Read the model definition and answer for the solid it produces. Units are mm, in the model's axes. Coordinates: 2 decimals unless noted, no trailing zeros. Write each loop counter-clockwise with the first axis right and the second up, starting at its lowest first coordinate (ties: lowest second). Pieces come first, ordered by that corner, then holes.
Item 1: Section C-C (z = -3.5) is taken. State how many separate pieces and enclosed holes the cut face has, then the cut area to 3 significant figures.
Item 2: Section B-B (y = -86.5) is taken. Give the vertices of the cut face in (x, z), then the cut area to 3 significant figures.
Item 3: Section A-A (x = 19) is taken. Give the vertices of the cut face in (y, z).
Item 4: Straight lines are drawn through the part: probe 1 along X at (y, z) = (-325, -0.25); probe 2 along Y at (x, z) = (475, -0.5); probe 3 along X at (y, z) = (-375, -1.5). For each, find the intervals that lie inside material, in ascending order.
Item 5: Each of these flat-tipped pins is pushed along its axis until it touches: P1, Ø3, axis at x = 466, z = 2, coming from the +Y side; P2, Ø3, axis at y = -371.5, z = -2, coming from the -X side; P3, Ø16.5, axis at x = -475, y = -325, coming from the +Z side; P4, Ø5, axis at y = 368.5, z = 0.5, coming from the +X side. Where does it stop, or does it pass through?
Autodesk Inventor part; units mm, degrees
ref_plane "YZ Plane" through (0, 0, 0) normal (1, 0, 0) x (0, 1, 0)
ref_plane "XZ Plane" through (0, 0, 0) normal (0, 1, 0) x (-1, 0, 0)
ref_plane "XY Plane" through (0, 0, 0) normal (0, 0, 1) x (1, 0, 0)
sketch "Sketch3" plane through (0, 0, 0) normal (0, 0, 1) x (1, 0, 0)
  line L0 (-500, -400) -> (500, -400)
  line L1 (500, -400) -> (500, 400)
  line L2 (500, 400) -> (-500, 400)
  line L3 (-500, 400) -> (-500, -400)
  line L4 (-500, -400) -> (500, 400) construction
  line L5 (500, -400) -> (-500, 400) construction
  point P0 (0, 0)
  dimension "d9" = 1000
  dimension "d10" = 800
extrude "Plate2" add sketch "Sketch3" along normal mid plane 10
sketch "Sketch4" plane through (0, 0, 5) normal (0, 0, 1) x (1, 0, 0)
  line L0 (-200, -175) -> (200, -175)
  line L1 (200, -175) -> (200, 175)
  line L2 (200, 175) -> (-200, 175)
  line L3 (-200, 175) -> (-200, -175)
  line L4 (-200, -175) -> (200, 175) construction
  line L5 (200, -175) -> (-200, 175) construction
  point P0 (0, 0)
  dimension "d12" = 400
  dimension "d13" = 350
extrude "Cut2" cut sketch "Sketch4" against normal blind 10
sketch "Sketch7" plane through (0, 0, 5) normal (0, 0, 1) x (1, 0, 0)
  line L0 (-450, 400) -> (-500, 400)
  line L1 (-500, 400) -> (-500, 350)
  line L2 (-500, 350) -> (-450, 350)
  line L3 (-450, 350) -> (-450, 400)
  line L4 (-450, 400) -> (-500, 350) construction
  line L5 (-500, 400) -> (-450, 350) construction
  circle A0 centre (-425, 375) radius 5.1
  circle A1 centre (-475, 325) radius 5.1
  point P0 (0, 0)
  point P1 (-475, 375)
  point P2 (-475, 375)
  point P3 (-475, 375)
  dimension "d20" = 50
  dimension "d21" = 50
  dimension "d26" = 10.2
  dimension "d27" = 25
  dimension "d28" = 25
extrude "Cut4" cut sketch "Sketch7" against normal blind 10
mirror "Mirror5" about plane through (0, 0, 0) normal (0, 1, 0) of "Cut4"
mirror "Mirror6" about plane through (0, 0, 0) normal (1, 0, 0) of "Cut4", "Mirror5"
equation "\"d14\" = Thickness"
equation "\"d21\" = d20"
equation "\"d28\" = d27"
equation "\"d22\" = Thickness"
equation "\"d11\" = Thickness"
equation "\"BendReliefDepth\" = 0.5 * Thickness"
properties part number "Chapa-0001-001" material "Steel, Galvanized"
Established:
1. separate pieces: 1
1. enclosed holes: 9
1. area: 649,000 mm2
2. outline: (-500, -5) - (-200, -5) - (-200, 5) - (-500, 5) - close; (200, -5) - (500, -5) - (500, 5) - (200, 5) - close
2. area: 6,000 mm2
3. outline: (-400, -5) - (-175, -5) - (-175, 5) - (-400, 5) - close; (175, -5) - (400, -5) - (400, 5) - (175, 5) - close
4. probe 1: x = -500 to -480.1, -469.9 to 469.9, 480.1 to 500
4. probe 2: y = -350 to -330.1, -319.9 to 319.9, 330.1 to 350
4. probe 3: x = -450 to -430.1, -419.9 to 419.9, 430.1 to 450
5. P1: stops at y = 350
5. P2: stops at x = -450
5. P3: stops at z = 5
5. P4: stops at x = 450
